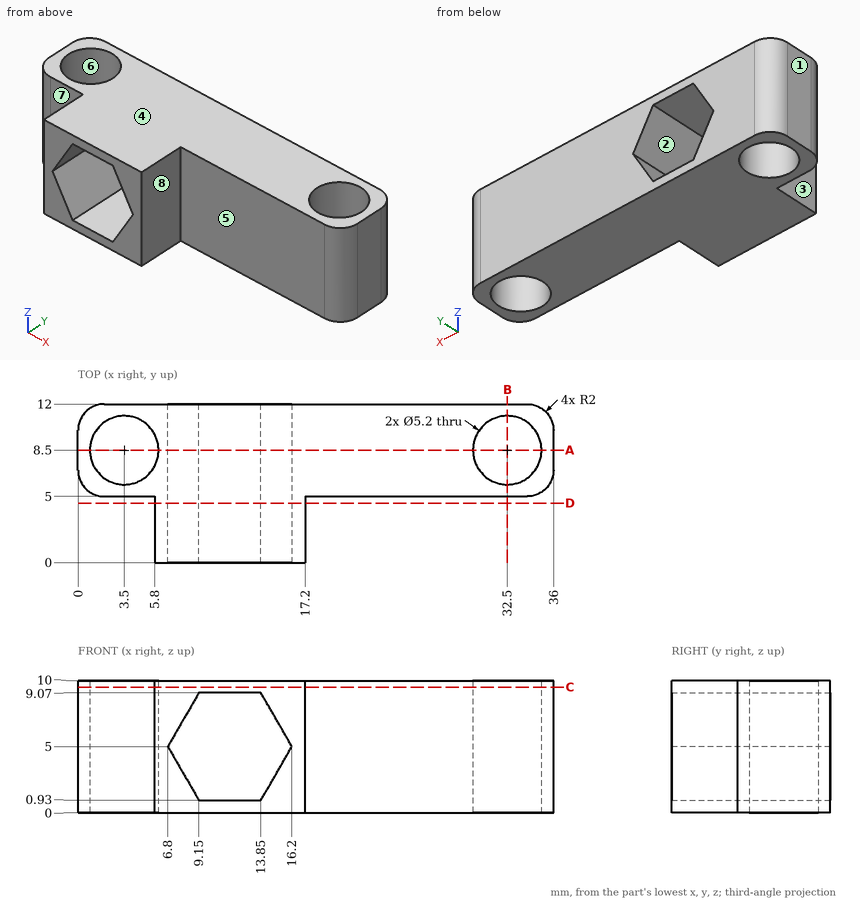
Part print with two shaded views. Sizes in mm from the minimum x, y, z corner. A direction names the side the tool comes from. Round coordinates to 2 decimals unless told otherwise and drop trailing zeros. Loops run counter-clockwise (first coordinate to the right, second up) from the corner with the lowest first, then second, coordinate; pieces in that order, holes last. Notation, with made-up numbers: (17, 45) - (40, 45) arc R16 cw to (40, 73) - close; hole circle Ø9 at (70, 26). An arc over 180 degrees is marked (long way). Put each result on its own line as item: value.
1. Slice it at C-C on z = 9.5. List the corners of the cut face in (x, y), and give its area (3 significant figures).
Geometry check:
outline: (0, 7) arc R2 ccw to (2, 5) - (5.8, 5) - (5.8, 0) - (17.2, 0) - (17.2, 5) - (34, 5) arc R2 ccw to (36, 7) - (36, 10) arc R2 ccw to (34, 12) - (2, 12) arc R2 ccw to (0, 10) - close; hole circle Ø5.2 at (3.5, 8.5); hole circle Ø5.2 at (32.5, 8.5)
area: 263 mm²
2. Slice it at D-D on y = 4.5. List the corners of the cut face in (x, z).
Geometry check:
outline: (5.8, 0) - (17.2, 0) - (17.2, 10) - (5.8, 10) - close; hole (6.8, 5) - (9.15, 0.93) - (13.85, 0.93) - (16.2, 5) - (13.85, 9.07) - (9.15, 9.07) - close
3. Slice it at B-B on x = 32.5. List the corners of the cut face in (y, z).
Geometry check:
outline: (5, 0) - (5.9, 0) - (5.9, 10) - (5, 10) - close; (11.1, 0) - (12, 0) - (12, 10) - (11.1, 10) - close
4. Wall check: line 1 (Y direction, x = 3.5, z = 4); line 2 (X direction, y = 7.5, z = 5.5); line 3 (Z direction, x = 9.5, y = 11.25). Give the ranges that are in metal, low to high.
Geometry check:
line 1: 5 to 5.9, 11.1 to 12
line 2: 0 to 1.1, 5.9 to 7.09, 15.91 to 30.1, 34.9 to 36
line 3: 0 to 0.93, 9.07 to 10
5. Slice it at A-A on y = 8.5. List the corners of the cut face in (x, z).
Geometry check:
outline: (0, 0) - (0.9, 0) - (0.9, 10) - (0, 10) - close; (6.1, 0) - (29.9, 0) - (29.9, 10) - (6.1, 10) - close; (35.1, 0) - (36, 0) - (36, 10) - (35.1, 10) - close; hole (6.8, 5) - (9.15, 0.93) - (13.85, 0.93) - (16.2, 5) - (13.85, 9.07) - (9.15, 9.07) - close
6. Pin check, flat tips, straight feed: P1, Ø2, axis at y = 4.5, z = 7.5, coming from the -X side; P2, Ø3, axis at x = 32.5, y = 8.5, coming from the +Z side; P3, Ø5.5, axis at y = 2, z = 4.5, coming from the -X side; P4, Ø5, axis at x = 28, z = 4.5, coming from the -Y side. Stop position of each tip, or through.
Geometry check:
P1: x = 0.68
P2: through
P3: x = 5.8
P4: y = 5
7. Two-plate mould, pull along X, no slides. Class the marked faces 6, 7 and 8: released by +X, released by -X, zero draft, split by the parting line, or undercut.
Geometry check:
face 6: undercut
face 7: zero draft
face 8: released by +X
8. 3-axis set-ups, long thin cutter, end or side, ignore diameter. For the marked faces 1, 2, 3, 4 and 5: which of +Z, -Z, +X, -X, +Y, -Y reach the whole face in a straight line?
Geometry check:
face 1: +Z, -Z, -X, +Y, -Y
face 2: +Y, -Y
face 3: +Z, -Z, -X, -Y
face 4: +Z, +X, -X, +Y, -Y
face 5: +Z, -Z, +X, -Y
